Model file for the job. Use its own axes, mm. Face numbers are marked on the shaded views. Round coordinates to 2 decimals unless told otherwise and drop trailing zeros. Order: outer loops, then holes, each group sorted by start corner. A loop starts at its lowest first (then second) coordinate and runs counter-clockwise, first axis right, second up. Notation, with made-up numbers: (-1.5, -20.5) - (32.5, -20.5) arc R15 cw to (32.5, 7.5) - close; hole circle Ø2 at (-12, -23). An arc over 180 degrees is marked (long way). Answer as CSV lines item,"result". Start each with the question number.
1. Band-saw the part on A-A on x = -18. List the corners of the cut face in (y, z), then the cut area to 3 significant figures.
2. Band-saw the part on B-B on y = 41.5. List the corners of the cut face in (x, z), then the cut area to 3 significant figures.
3. Pin check, flat tips, straight feed: pin 1 Ø2 at (x, z) = (25, 0.5) entering from -Y; pin 2 Ø3.5 at (x, y) = (41, -1) entering from +Z; pin 3 Ø1.5 at (y, z) = (32, 2) entering from +X; pin 4 Ø1.9 at (x, y) = (41.275, 57.6) entering from +Z. Stop position of each tip, or through.
4. Wall check: line 1 along X through (y, z) = (8.55, -0.2); line 2 along Y through (x, z) = (36.5, 0.35); line 3 along Y through (x, z) = (-30, 0.15). Give the ranges that are in metal, low to high. Write a range as [from, to].
5. Pull direction Y, two halves, no side cores. Call the marked faces 1 and 2: released by +Y, released by -Y, zero draft, split by the parting line, or undercut.
```python
from build123d import *

# Parameters (mm, degrees)
BOSS_EXTRUDE1_DEPTH                            = 3
BOSS_EXTRUDE4_START                            = 1.5
SKETCH5_R                                      = 2.5
BOSS_EXTRUDE4_DEPTH                            = 1.5
SKETCH3_R                                      = 1.2
CUT_EXTRUDE1_DEPTH                             = 75.488325428
CUT_EXTRUDE2_START                             = -1
CUT_EXTRUDE2_DEPTH                             = 1
BOSS_EXTRUDE6_START                            = 3
SKETCH8_R                                      = 3
BOSS_EXTRUDE6_DEPTH                            = 3
CSK_FOR_M2_FLAT_HEAD_MACHINE_SCREW1_AT_2_COUNT = 2
CSK_FOR_M2_FLAT_HEAD_MACHINE_SCREW1_AT_2_PITCH = 69.354163538


with BuildPart() as part:
    # Sketch1 → Boss-Extrude1 (new body)
    with BuildSketch(Plane.XY):
        with BuildLine():
            Line((-39.803551907, 59.621098837), (-30.752483537, 53.031526348))
            Line((-30.752483537, 53.031526348), (30.752483537, 53.031526348))
            Line((30.752483537, 53.031526348), (39.803551907, 59.621098837))
            ThreePointArc((39.803551907, 59.621098837), (43.296098837, 59.071448093), (42.746448093, 55.578901163))
            Line((42.746448093, 55.578901163), (35, 49.939149129))
            Line((35, 49.939149129), (35, 18.55))
            Line((35, 18.55), (39, 18.55))
            ThreePointArc((39, 18.55), (42, 15.55), (39, 12.55))
            Line((39, 12.55), (35, 12.55))
            Line((35, 12.55), (35, 5.160850871))
            Line((35, 5.160850871), (42.746448093, -0.478901163))
            ThreePointArc((42.746448093, -0.478901163), (43.296098837, -3.971448093), (39.803551907, -4.521098837))
            Line((39.803551907, -4.521098837), (30.752483537, 2.068473652))
            Line((30.752483537, 2.068473652), (-30.752483537, 2.068473652))
            Line((-30.752483537, 2.068473652), (-39.803551907, -4.521098837))
            ThreePointArc((-39.803551907, -4.521098837), (-43.296098837, -3.971448093), (-42.746448093, -0.478901163))
            Line((-42.746448093, -0.478901163), (-35, 5.160850871))
            Line((-35, 5.160850871), (-35, 49.939149129))
            Line((-35, 49.939149129), (-42.746448093, 55.578901163))
            ThreePointArc((-42.746448093, 55.578901163), (-43.296098837, 59.071448093), (-39.803551907, 59.621098837))
        make_face()
    extrude(amount=BOSS_EXTRUDE1_DEPTH)

    # Sketch5 → Boss-Extrude4 (add)
    with BuildSketch(Plane(origin=(0, 0, 0), x_dir=(-1, 0, 0), z_dir=(0, 0, -1)).offset(BOSS_EXTRUDE4_START)):
        with Locations((-41.275, 57.6)):
            Circle(SKETCH5_R)
        with Locations((41.275, 57.6)):
            Circle(SKETCH5_R)
        with Locations((-41.275, -2.5)):
            Circle(SKETCH5_R)
        with Locations((41.275, -2.5)):
            Circle(SKETCH5_R)
    extrude(amount=-BOSS_EXTRUDE4_DEPTH)

    # Sketch3 → Cut-Extrude1 (cut, through all)
    with BuildSketch(Plane.XY.offset(3)):
        with Locations((-41.275, 57.6)):
            Circle(SKETCH3_R)
        with Locations((41.275, 57.6)):
            Circle(SKETCH3_R)
        with Locations((-41.275, -2.5)):
            Circle(SKETCH3_R)
        with Locations((41.275, -2.5)):
            Circle(SKETCH3_R)
    extrude(amount=-CUT_EXTRUDE1_DEPTH, mode=Mode.SUBTRACT)

    # Sketch7 → Cut-Extrude2 (cut)
    with BuildSketch(Plane.XY.offset(3).offset(CUT_EXTRUDE2_START)):
        with BuildLine():
            Line((-36.569793768, 57.266781888), (-39.512689954, 53.224584214))
            Line((-39.512689954, 53.224584214), (-42.746448093, 55.578901163))
            ThreePointArc((-42.746448093, 55.578901163), (-43.296098837, 59.071448093), (-39.803551907, 59.621098837))
            Line((-39.803551907, 59.621098837), (-36.569793768, 57.266781888))
        make_face()
        with BuildLine():
            Line((-42.746448093, -0.478901163), (-39.512689954, 1.875415786))
            Line((-39.512689954, 1.875415786), (-36.569793768, -2.166781888))
            Line((-36.569793768, -2.166781888), (-39.803551907, -4.521098837))
            ThreePointArc((-39.803551907, -4.521098837), (-43.296098837, -3.971448093), (-42.746448093, -0.478901163))
        make_face()
        with BuildLine():
            Line((39.803551907, -4.521098837), (36.569793768, -2.166781888))
            Line((36.569793768, -2.166781888), (39.512689954, 1.875415786))
            Line((39.512689954, 1.875415786), (42.746448093, -0.478901163))
            ThreePointArc((42.746448093, -0.478901163), (43.296098837, -3.971448093), (39.803551907, -4.521098837))
        make_face()
        with BuildLine():
            Line((39.803551907, 59.621098837), (36.569793768, 57.266781888))
            Line((36.569793768, 57.266781888), (39.512689954, 53.224584214))
            Line((39.512689954, 53.224584214), (42.746448093, 55.578901163))
            ThreePointArc((42.746448093, 55.578901163), (43.296098837, 59.071448093), (39.803551907, 59.621098837))
        make_face()
    extrude(amount=CUT_EXTRUDE2_DEPTH, mode=Mode.SUBTRACT)

    # Sketch8 → Boss-Extrude6 (add)
    with BuildSketch(Plane(origin=(0, 0, 0), x_dir=(-1, 0, 0), z_dir=(0, 0, -1)).offset(BOSS_EXTRUDE6_START)):
        with Locations((-39, 15.55)):
            Circle(SKETCH8_R)
        with Locations(Location((30, 8.55, 0), (0, 0, 180))):
            Circle(SKETCH8_R)
    extrude(amount=-BOSS_EXTRUDE6_DEPTH)

    # Sketch11 → CSK for M2 Flat Head Machine Screw1 (revolve, cut)
    with BuildSketch(Plane(origin=(39, 15.55, -3), x_dir=(0, 1, 0), z_dir=(1, 0, 0))):
        Polygon((0, 0), (0, 4.901290929), (1.5, 4), (1.5, 0.503826859), (1.635, 0), align=None)
    csk_for_m2_flat_head_machine_screw1 = revolve(axis=Axis((39, 15.55, -9.35), (0, 0, 1)), mode=Mode.SUBTRACT)

    # CSK for M2 Flat Head Machine Screw1 at 2: CSK for M2 Flat Head Machine Screw1 ×2
    with Locations(*[Vector(-0.9948934062566149, -0.10093121512748267, 0) * (i * CSK_FOR_M2_FLAT_HEAD_MACHINE_SCREW1_AT_2_PITCH) for i in range(1, CSK_FOR_M2_FLAT_HEAD_MACHINE_SCREW1_AT_2_COUNT)]):
        add(csk_for_m2_flat_head_machine_screw1, mode=Mode.SUBTRACT)


solid = part.part
```
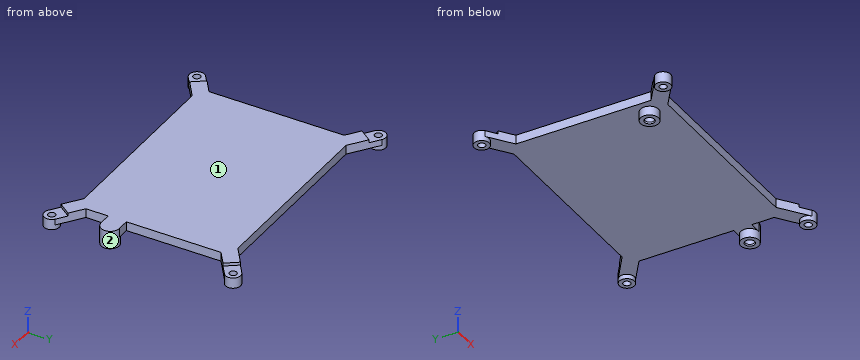
Reply:
1,outline,"(2.07, 0) - (53.03, 0) - (53.03, 3) - (2.07, 3) - close"
1,area,"153 mm2"
2,outline,"(-35, 0) - (35, 0) - (35, 3) - (-35, 3) - close"
2,area,"210 mm2"
3,pin 1,"stops at y = 2.07"
3,pin 2,"stops at z = 2"
3,pin 3,"stops at x = 35"
3,pin 4,"passes through"
4,line 1,"x = [-33, -31.5], [-28.5, -27]"
4,line 2,"y = [-2.12, 4.07], [12.55, 18.55], [51.03, 57.22]"
4,line 3,"y = [2.07, 7.05], [10.05, 53.03]"
5,face 1,"zero draft"
5,face 2,"undercut"
